from build123d import *
from OCP.BRepFilletAPI import BRepFilletAPI_MakeChamfer

# Parameters (mm, degrees)
BOSS_EXTRUDE1_DEPTH = 166.66666666666666
CUT_EXTRUDE1_DEPTH  = 160.666666667
BOSS_EXTRUDE2_DEPTH = 4
SKETCH9_R           = 2.1999999999999833
CUT_EXTRUDE3_DEPTH  = 673.8557295952264
SKETCH10_R          = 2.1999999999999833
CUT_EXTRUDE4_DEPTH  = 3
CHAMFER3_SIZE       = 0.6
CHAMFER3_SIZE2      = 0.5047874406768073
CHAMFER4_SIZE       = 1
CHAMFER4_SIZE2      = 0.8287182147663876
CHAMFER8_SIZE       = 4
CHAMFER9_SIZE       = 4


with BuildPart() as part:
    # Sketch4 → Boss-Extrude1 (new body)
    with BuildSketch(Plane.XY):
        Polygon((-500.7204776760873, 35.989612544106855), (-649.8557297792629, -1.837e-14), (-499.8557297792629, -6.121e-14), align=None)
    extrude(amount=-BOSS_EXTRUDE1_DEPTH)

    # Sketch6 → Cut-Extrude1 (cut)
    with BuildSketch(Plane.XY.offset(-3)):
        Polygon((-504.85717289786834, -1.837e-14), (-505.570212772658, 29.675734299461347), (-585.1090138943516, 10.481274275937695), (-584.8571728978683, -1.837e-14), align=None)
    extrude(amount=-CUT_EXTRUDE1_DEPTH, mode=Mode.SUBTRACT)

    # Sketch8 → Boss-Extrude2 (add)
    with BuildSketch(Plane.XY):
        Polygon((-500.3361452774986, 19.994229191170454), (-470.34480149074295, 20.714852438524037), (-469.86438599250715, 0.720623247353527), (-499.8557297792629, -6.121e-14), (-529.8643884908956, -2.204e-14), (-530.3274890642546, 19.273605943816776), align=None)
    extrude(amount=BOSS_EXTRUDE2_DEPTH)

    # Sketch9 → Cut-Extrude3 (cut, through all)
    with BuildSketch(Plane.XY.offset(4)):
        with Locations((-485.1002656350029, 10.357426219261987)):
            Circle(SKETCH9_R)
    extrude(amount=-CUT_EXTRUDE3_DEPTH, mode=Mode.SUBTRACT)

    # Sketch10 → Cut-Extrude4 (cut)
    with BuildSketch(Plane(origin=(0, 0, -166.66666666666666), x_dir=(-1, 0, 0), z_dir=(0, 0, -1))):
        with Locations((513.1478143821638, 11.99999999999998)):
            Circle(SKETCH10_R)
        with Locations((527.1478143821638, 11.99999999999998)):
            Circle(SKETCH10_R)
    extrude(amount=-CUT_EXTRUDE4_DEPTH, mode=Mode.SUBTRACT)

    # Chamfer3: one chamfer whose edges measure the first distance from different faces: ONE call of the kernel's chamfer builder (chamfer() names one face for all edges)
    chamfer3_edges_1 = [part.edges().sort_by_distance(p)[0] for p in [
        (-500.7204776760873, 35.989612544106855, -83.33333333333333),
    ]]
    chamfer3_side_1 = [part.faces().sort_by_distance(p)[0] for p in [
        (-575.2881037276751, 17.994806272053417, -83.33333333333333),
    ]]
    chamfer3_edges_2 = [part.edges().sort_by_distance(p)[0] for p in [
        (-575.2881037276751, 17.994806272053417, -166.66666666666666),
    ]]
    chamfer3 = BRepFilletAPI_MakeChamfer(part.part.solid().wrapped)
    for e in chamfer3_edges_1:
        chamfer3.Add(CHAMFER3_SIZE, CHAMFER3_SIZE2, e.wrapped, chamfer3_side_1[0].wrapped)  # the first distance lies on this face
    for e in chamfer3_edges_2:
        chamfer3.Add(CHAMFER3_SIZE, e.wrapped)
    add(Compound.cast(chamfer3.Shape()), mode=Mode.REPLACE)

    # Chamfer4
    chamfer4_edges = [part.edges().sort_by_distance(p)[0] for p in [
        (-649.8557297792629, -1.837e-14, -83.03333333333336),
    ]]
    chamfer4_side = [part.faces().sort_by_distance(p)[0] for p in [
        (-605.6991208479849, -3.098e-14, -82.49305945140193),
    ]]
    chamfer(chamfer4_edges, length=CHAMFER4_SIZE, length2=CHAMFER4_SIZE2, reference=chamfer4_side[0])

    # Chamfer8
    chamfer8_edges = [part.edges().sort_by_distance(p)[0] for p in [
        (-515.3318171708765, 19.633917567493594, 0),
    ]]
    chamfer(chamfer8_edges, length=CHAMFER8_SIZE - 0.0001)  # a hair under: the kernel refuses the full size

    # Chamfer9
    chamfer9_edges = [part.edges().sort_by_distance(p)[0] for p in [
        (-530.1439791263599, 11.636175905452475, 0),
    ]]
    chamfer(chamfer9_edges, length=CHAMFER9_SIZE - 0.0001)  # a hair under: the kernel refuses the full size


solid = part.part
Can you work these out from the model? Positions are in its coordinate system, mm. A direction names the side the tool comes from. Give positions to 0.01 mm unless a question says otherwise; leave off trailing zeros. Write each loop counter-clockwise with the first axis right and the second up, starting at its lowest first coordinate (ties: lowest second). Pieces come first, ordered by that corner, then holes. Notation, with made-up numbers: M -22.5,38.25 L -9.5,38.25 A14 cw -9.5,50.25 Z; hole C -7.5,-20.5 d4. An arc over 180 degrees is marked long. Answer in a Markdown table with one row per item. Add a question column.
Item 1: We'd pull the mould along Z, two halves only. Please class faces 3 (the cylindrical face through (-510.95, 12.1, -165.19)), 4 (the flat face through (-564, 14, 0)), 5 (the flat face through (-537, 12, -163.667)), 6 (the flat face through (-537, 12, -3)): released by +Z, released by -Z, zero draft, split by the parting line, or undercut.
Item 2: Please list where these lines run through material, in increasing order: L1, parallel to Z at x = -558.5, y = 7; L2, parallel to Z at x = -519.5, y = 20; L3, parallel to Z at x = -486.5, y = 5.5.
Item 3: For pin 1 Ø5 at (y, z) = (11.5, -16) entering from +X; pin 2 Ø18 at (x, y) = (-574.5, 13.5) entering from +Z; pin 3 Ø4 at (x, y) = (-513.15, 12) entering from -Z; pin 4 Ø3 at (x, y) = (-492.5, 22.5) entering from -Z, each with a flat end and sliding along its axis, tell me the tip position at first contact or that it passes through.
Item 4: On a 3-axis mill with a long thin cutter (end or side, diameter ignored), from which of +Z, -Z, +X, -X, +Y, -Y can I reach the whole of each face in a straight line? I mean faces 1 (the cylindrical face through (-487.3, 10.45, 2.03)), 2 (the cylindrical face through (-524.95, 12.1, -165.19)). Say none if no direction works.
Item 5: Imagine slicing it at A-A, the plane z = -52.5. Write out the boundary of the cut face in (x, y), plus the area to 3 significant figures.
Item 6: Imagine slicing it at B-B, the plane x = -552. Write out the boundary of the cut face in (y, z), plus the area to 3 significant figures.
Evaluation:
| question | item | result |
|---|---|---|
| 1 | face 3 | zero draft |
| 1 | face 4 | released by +Z |
| 1 | face 5 | undercut |
| 1 | face 6 | undercut |
| 2 | L1 | z = -166.67 to -163.67, -3 to 0 |
| 2 | L2 | z = -166.67 to -163.67, -3 to 3.53 |
| 2 | L3 | z = 0 to 4 |
| 3 | pin 1 | stops at x = -500.07 |
| 3 | pin 2 | stops at z = 0 |
| 3 | pin 3 | stops at z = -3 |
| 3 | pin 4 | passes through |
| 4 | face 1 | +Z, -Z |
| 4 | face 2 | -Z |
| 5 | outline | M -649.05,0.19 L -648.86,0 L -584.86,0 L -585.11,10.48 L -505.57,29.68 L -504.86,0 L -499.86,0 L -500.71,35.48 L -501.3,35.85 Z |
| 5 | area | 1,090 mm² |
| 6 | outline | M 0,-166.67 L 23,-166.67 L 23.61,-166.07 L 23.61,0 L 0,0 L 0,-3 L 18.47,-3 L 18.47,-163.67 L 0,-163.67 Z |
| 6 | area | 968 mm² |
